Read the model definition and answer for the solid it produces. Units are mm, in the model's axes. Face numbers are marked on the shaded views. A direction names the side the tool comes from. Round coordinates to 2 decimals unless told otherwise and drop trailing zeros. Order: outer loops, then holes, each group sorted by start corner. A loop starts at its lowest first (then second) coordinate and runs counter-clockwise, first axis right, second up. Notation, with made-up numbers: (36.5, 42) -> (68.5, 42) arc R13 cw to (68.5, 63) -> close; hole circle Ø10 at (0.25, 82.25). An arc over 180 degrees is marked (long way). Answer as a JSON object with one key per item and string values. Group by question number.
Item 1: Consider probe 1 along Y at (x, z) = (77.5, 0.9); probe 2 along Y at (x, z) = (13.08, 0.5); probe 3 along Y at (x, z) = (16, 7.5). Determine where each line is inside the solid, lowest interval first. Write a range as from..to.
Item 2: For the marked faces 1, 2, 3, 4 and 5, determine the directions among +Z, -Z, +X, -X, +Y, -Y from which every point of the face is accessible in a straight line to the end or side of a thin tool.
Item 3: Section A-A, the plane x = 2.5 is taken. Write down the section's boundary in (y, z), plus the area to 3 significant figures.
Item 4: Section B-B, the plane x = 53.5 is taken. Write down the section's boundary in (y, z).
Item 5: Section D-D, the plane z = 6.75 is taken. Write down the section's boundary in (x, y), plus the area to 3 significant figures.
Item 6: Section C-C, the plane y = 26 is taken. Write down the section's boundary in (x, z), plus the area to 3 significant figures.
Item 7: Given P1, Ø1.5, axis at x = 62.5, z = 2.5, coming from the -Y side; P2, Ø5, axis at y = 20, z = 9, coming from the -X side; P3, Ø3, axis at x = 40.5, y = 26, coming from the -Z side; P4, Ø3, axis at x = 77.5, y = 33.5, coming from the +Z side, each flat-ended and moving along its own axis, determine where each tip first touches the part or whether it passes through.
from build123d import *

# Parameters (mm, degrees)
ESBO_O1_W                = 80
ESBO_O1_H                = 36
ESBO_O1_R                = 1.35
RESSALTO_EXTRUS_O1_DEPTH = 1.6
ESBO_O4_W                = 65.5
ESBO_O4_H                = 14.5
RESSALTO_EXTRUS_O2_DEPTH = 9.6
ESBO_O3_W                = 72.2
ESBO_O3_H                = 24.1
RESSALTO_EXTRUS_O3_DEPTH = 9.5
ESBO_O5_R                = 0.5
CORTE_EXTRUS_O1_DEPTH    = 2.6


with BuildPart() as part:
    # Esboço1 → Ressalto-extrusão1 (new body)
    with BuildSketch(Plane.XY):
        with Locations((40, 18)):
            Rectangle(ESBO_O1_W, ESBO_O1_H)
        with Locations((2.5, 33.5)):
            Circle(ESBO_O1_R, mode=Mode.SUBTRACT)
        with Locations((2.5, 2.5)):
            Circle(ESBO_O1_R, mode=Mode.SUBTRACT)
        with Locations((77.5, 33.5)):
            Circle(ESBO_O1_R, mode=Mode.SUBTRACT)
        with Locations((77.5, 2.5)):
            Circle(ESBO_O1_R, mode=Mode.SUBTRACT)
    extrude(amount=RESSALTO_EXTRUS_O1_DEPTH)

    # Esboço4 → Ressalto-extrusão2 (add)
    with BuildSketch(Plane.XY.offset(1.6)):
        with Locations((40, 18)):
            Rectangle(ESBO_O4_W, ESBO_O4_H)
    extrude(amount=RESSALTO_EXTRUS_O2_DEPTH)

    # Esboço3 → Ressalto-extrusão3 (add)
    with BuildSketch(Plane.XY.offset(1.6)):
        with Locations((40, 17.85)):
            Rectangle(ESBO_O3_W, ESBO_O3_H)
    extrude(amount=RESSALTO_EXTRUS_O3_DEPTH)

    # Esboço5 → Corte-extrusão1 (cut, through all)
    with BuildSketch(Plane.XY.offset(1.6)):
        with Locations((8, 33.5)):
            Circle(ESBO_O5_R)
        with Locations((10.54, 33.5)):
            Circle(ESBO_O5_R)
        with Locations((13.08, 33.5)):
            Circle(ESBO_O5_R)
        with Locations((15.62, 33.5)):
            Circle(ESBO_O5_R)
        with Locations((18.16, 33.5)):
            Circle(ESBO_O5_R)
        with Locations((20.7, 33.5)):
            Circle(ESBO_O5_R)
        with Locations((23.24, 33.5)):
            Circle(ESBO_O5_R)
        with Locations((25.78, 33.5)):
            Circle(ESBO_O5_R)
        with Locations((28.32, 33.5)):
            Circle(ESBO_O5_R)
        with Locations((30.86, 33.5)):
            Circle(ESBO_O5_R)
        with Locations((33.4, 33.5)):
            Circle(ESBO_O5_R)
        with Locations((35.94, 33.5)):
            Circle(ESBO_O5_R)
        with Locations((38.48, 33.5)):
            Circle(ESBO_O5_R)
        with Locations((41.02, 33.5)):
            Circle(ESBO_O5_R)
        with Locations((43.56, 33.5)):
            Circle(ESBO_O5_R)
        with Locations((46.1, 33.5)):
            Circle(ESBO_O5_R)
    extrude(amount=-CORTE_EXTRUS_O1_DEPTH, mode=Mode.SUBTRACT)


solid = part.part
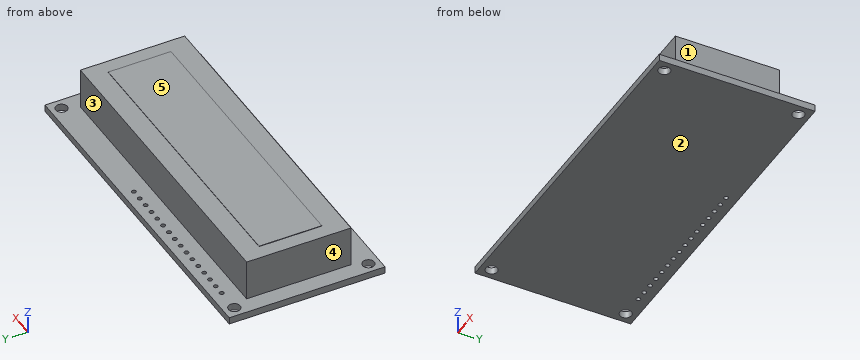
Values found:
{
 "1": {"probe 1": "0..1.15, 3.85..32.15, 34.85..36", "probe 2": "0..33, 34..36", "probe 3": "5.8..29.9"},
 "2": {"face 1": "+Z, +X, +Y, -Y", "face 2": "-Z, +X, -X, +Y, -Y", "face 3": "+Z, +X, -X, +Y", "face 4": "+Z, -X, +Y, -Y", "face 5": "+Z, +X, -X, +Y, -Y"},
 "3": {"outline": "(0, 0) -> (1.15, 0) -> (1.15, 1.6) -> (0, 1.6) -> close; (3.85, 0) -> (32.15, 0) -> (32.15, 1.6) -> (3.85, 1.6) -> close; (34.85, 0) -> (36, 0) -> (36, 1.6) -> (34.85, 1.6) -> close", "area": "49.0 mm2"},
 "4": {"outline": "(0, 0) -> (36, 0) -> (36, 1.6) -> (29.9, 1.6) -> (29.9, 11.1) -> (25.25, 11.1) -> (25.25, 11.2) -> (10.75, 11.2) -> (10.75, 11.1) -> (5.8, 11.1) -> (5.8, 1.6) -> (0, 1.6) -> close"},
 "5": {"outline": "(3.9, 5.8) -> (76.1, 5.8) -> (76.1, 29.9) -> (3.9, 29.9) -> close", "area": "1,740 mm2"},
 "6": {"outline": "(0, 0) -> (80, 0) -> (80, 1.6) -> (76.1, 1.6) -> (76.1, 11.1) -> (3.9, 11.1) -> (3.9, 1.6) -> (0, 1.6) -> close", "area": "814 mm2"},
 "7": {"P1": "y = 5.8", "P2": "x = 3.9", "P3": "z = 0", "P4": "z = 1.6"}
}
